Check sheet for the modelled part. Datum: model origin and axes. Units: mm. A direction names the side the tool comes from. Give positions to 0.01 mm unless a question says otherwise; leave off trailing zeros. Order: outer loops, then holes, each group sorted by start corner. A loop starts at its lowest first (then second) coordinate and runs counter-clockwise, first axis right, second up. Notation, with made-up numbers: (-24.5, 4.25) -> (-13.5, 4.25) arc R27 cw to (-13.5, 26.25) -> close; hole circle Ø10 at (-11, 29). An arc over 180 degrees is marked (long way). Write each question's results on one line, items separated by ' | '.
from build123d import *

# Parameters (mm, degrees)
SALIENTE_EXTRUIR1_DEPTH = 10


with BuildPart() as part:
    # Croquis1 → Saliente-Extruir1 (new body)
    with BuildSketch(Plane.XY):
        with BuildLine():
            Line((37.91601702, 121.421613069), (114.537816123, 144.025264418))
            ThreePointArc((114.537816123, 144.025264418), (127.193827362, 151.843476845), (134.121677329, 165.007973069))
            ThreePointArc((134.121677329, 165.007973069), (132.264993157, 210.622251423), (102.682371845, 245.392614983))
            ThreePointArc((102.682371845, 245.392614983), (95.369412387, 253.859995337), (94.665863515, 265.026056643))
            Line((94.665863515, 265.026056643), (107.60681577, 313.322347957))
            ThreePointArc((107.60681577, 313.322347957), (115.776254029, 323.968967178), (129.081215867, 325.720598634))
            Line((129.081215867, 325.720598634), (240, 296))
            Line((240, 296), (240, 0))
            Line((240, 0), (-0.665441115, -0.303814753))
            Line((-0.665441115, -0.303814753), (-0.665441115, 69.814722685))
            ThreePointArc((-0.665441115, 69.814722685), (10.046152069, 102.031954282), (37.91601702, 121.421613069))
        make_face()
    extrude(amount=SALIENTE_EXTRUIR1_DEPTH)


solid = part.part
1. Access from +Z, -Z, +X, -X, +Y, -Y to the whole of each face (thin tool, end or side, straight path). Record for faces 1 (the cylindrical face through (127.05, 151.69, 4.93)), 2 (the cylindrical face through (9.758, 101.643, 4.93)).
Verdict:
face 1: +Z, -Z, -X | face 2: +Z, -Z, -X, +Y
2. Material ranges on probe 1 along X at (y, z) = (89.5, 4); probe 2 along X at (y, z) = (105, 2.25); probe 3 along Y at (x, z) = (55.5, 3), recorded low to high. Write a range as from..to.
Verdict:
probe 1: x = 3.06..240 | probe 2: x = 12.43..240 | probe 3: y = -0.23..126.61
3. Section check B-B on y = 292. Record the cut outline in (x, z), then the cut area to 3 significant figures.
Verdict:
outline: (101.89, 0) -> (240, 0) -> (240, 10) -> (101.89, 10) -> close | area: 1,380 mm^2
4. Section check A-A on z = 5.75. Record the cut outline in (x, y), then the cut area to 3 significant figures.
Verdict:
outline: (-0.67, -0.3) -> (240, 0) -> (240, 296) -> (129.08, 325.72) arc R17.53 ccw to (107.61, 313.32) -> (94.67, 265.03) arc R17.53 ccw to (102.68, 245.39) arc R70 cw to (134.12, 165.01) arc R28.24 cw to (114.54, 144.03) -> (37.92, 121.42) arc R53.81 ccw to (-0.67, 69.81) -> close | area: 53,200 mm^2
5. Gauge pin test, flat ends, axial feed: pin 1 Ø2 at (y, z) = (292.5, 2) entering from -X; pin 2 Ø2 at (y, z) = (73, 4.5) entering from -X. Record the tip position at first contact, or that the pin passes through.
Verdict:
pin 1: stops at x = 101.76 | pin 2: stops at x = -0.62
6. Section check C-C on x = 160.5. Record the cut outline in (y, z), then the cut area to 3 significant figures.
Verdict:
outline: (-0.1, 0) -> (317.3, 0) -> (317.3, 10) -> (-0.1, 10) -> close | area: 3,170 mm^2
7. Mould release check, pull along Y, two halves, no side actions. Record for faces 3 (the flat face through (148, 129, 0)), 4 (the flat face through (75.691, 132.565, 4.93)), 5 (the flat face through (101.046, 288.836, 4.93)): +Y half, -Y half, draft (parallel to the pull), parting line (faces both ways), or undercut.
Verdict:
face 3: draft | face 4: undercut | face 5: +Y half
